Work out the finished part from the listing and answer in its coordinate system (mm). A direction names the side the tool comes from. Round coordinates to 2 decimals unless told otherwise and drop trailing zeros. Loops run counter-clockwise (first coordinate to the right, second up) from the corner with the lowest first, then second, coordinate; pieces in that order, holes last.
```python
from build123d import *

# Parameters (mm, degrees)
BOSS_EXTRUDE1_DEPTH = 12
CUT_EXTRUDE1_REACH  = 94.569
SKETCH2_R           = 3


with BuildPart() as part:
    # Sketch1 → Boss-Extrude1 (new body)
    with BuildSketch(Plane(origin=(0, 0, 0), x_dir=(1, 0, 0), z_dir=(0, 1, 0))):
        Polygon((-30, -30), (-45, -45), (-45, -80), (45, -80), (45, -45), (30, -30), (30, 30), (-30, 30), align=None)
    extrude(amount=BOSS_EXTRUDE1_DEPTH)

    # Sketch2 → Cut-Extrude1 (cut, up to next)
    with BuildSketch(Plane(origin=(0, 12, 0), x_dir=(1, 0, 0), z_dir=(0, 1, 0)), mode=Mode.PRIVATE) as cut_extrude1_sk1:
        with Locations(Location((-24, 20, 0), (0, 0, 270))):
            Circle(SKETCH2_R)
    cut_extrude1_tool1 = extrude(cut_extrude1_sk1.sketch, amount=-CUT_EXTRUDE1_REACH, mode=Mode.PRIVATE) & part.part
    # Sketch2 → Cut-Extrude1 (cut, up to next)
    with BuildSketch(Plane(origin=(0, 12, 0), x_dir=(1, 0, 0), z_dir=(0, 1, 0)), mode=Mode.PRIVATE) as cut_extrude1_sk2:
        with Locations(Location((-24, -20, 0), (0, 0, 270))):
            Circle(SKETCH2_R)
    cut_extrude1_tool2 = extrude(cut_extrude1_sk2.sketch, amount=-CUT_EXTRUDE1_REACH, mode=Mode.PRIVATE) & part.part
    # Sketch2 → Cut-Extrude1 (cut, up to next)
    with BuildSketch(Plane(origin=(0, 12, 0), x_dir=(1, 0, 0), z_dir=(0, 1, 0)), mode=Mode.PRIVATE) as cut_extrude1_sk3:
        with Locations(Location((24, 20, 0), (0, 0, 270))):
            Circle(SKETCH2_R)
    cut_extrude1_tool3 = extrude(cut_extrude1_sk3.sketch, amount=-CUT_EXTRUDE1_REACH, mode=Mode.PRIVATE) & part.part
    # Sketch2 → Cut-Extrude1 (cut, up to next)
    with BuildSketch(Plane(origin=(0, 12, 0), x_dir=(1, 0, 0), z_dir=(0, 1, 0)), mode=Mode.PRIVATE) as cut_extrude1_sk4:
        with Locations(Location((24, -20, 0), (0, 0, 270))):
            Circle(SKETCH2_R)
    cut_extrude1_tool4 = extrude(cut_extrude1_sk4.sketch, amount=-CUT_EXTRUDE1_REACH, mode=Mode.PRIVATE) & part.part
    add(cut_extrude1_tool1.solids().sort_by_distance((-24, 12, -20))[0], mode=Mode.SUBTRACT)
    add(cut_extrude1_tool2.solids().sort_by_distance((-24, 12, 20))[0], mode=Mode.SUBTRACT)
    add(cut_extrude1_tool3.solids().sort_by_distance((24, 12, -20))[0], mode=Mode.SUBTRACT)
    add(cut_extrude1_tool4.solids().sort_by_distance((24, 12, 20))[0], mode=Mode.SUBTRACT)


solid = part.part
```
1. Find section D-D (z = -9). Write down the section's boundary in (x, y), then the cut area to 3 significant figures.
Answer key:
outline: (-30, 0) - (30, 0) - (30, 12) - (-30, 12) - close
area: 720 mm2
2. Find section B-B (x = 24). Write down the section's boundary in (y, z).
Answer key:
outline: (0, -30) - (12, -30) - (12, -23) - (0, -23) - close; (0, -17) - (12, -17) - (12, 17) - (0, 17) - close; (0, 23) - (12, 23) - (12, 80) - (0, 80) - close
3. Find section C-C (z = -20). Write down the section's boundary in (x, y).
Answer key:
outline: (-30, 0) - (-27, 0) - (-27, 12) - (-30, 12) - close; (-21, 0) - (21, 0) - (21, 12) - (-21, 12) - close; (27, 0) - (30, 0) - (30, 12) - (27, 12) - close
4. Determine the mould class of faces 3 (the face through (-24, 6, -23)), 4 (the face through (-1, 0, 24)), 5 (the face through (30, 6, 0)), 6 (the face through (-37, 6, 37)) for opening direction X: +X half, -X half, draft (parallel to the pull), parting line (faces both ways), or undercut.
Answer key:
face 3: undercut
face 4: draft
face 5: +X half
face 6: -X half
5. Given pin 1 (4 mm diameter, centred on x = 34.5, y = 2.5, fed in from -Z); pin 2 (3.5 mm diameter, centred on y = 6.5, z = -0.5, fed in from +X); pin 3 (3 mm diameter, centred on x = 31, z = 0, fed in from +Y), each flat-ended and moving along its own axis, determine where each tip first touches the part or whether it passes through.
Answer key:
pin 1: stops at z = 32.5
pin 2: stops at x = 30
pin 3: stops at y = 12
6. Which of the six approach directions +Z, -Z, +X, -X, +Y, -Y give full straight-line access (tool end or side, diameter ignored) to faces 1 (the face through (-24, 6, 17)), 2 (the face through (-30, 6, 0))?
Answer key:
face 1: +Y, -Y
face 2: -Z, -X, +Y, -Y
7. Find section A-A (y = 7.5). Write down the section's boundary in (x, z), then the cut area to 3 significant figures.
Answer key:
outline: (-45, 45) - (-30, 30) - (-30, -30) - (30, -30) - (30, 30) - (45, 45) - (45, 80) - (-45, 80) - close; hole circle Ø6 at (-24, -20); hole circle Ø6 at (-24, 20); hole circle Ø6 at (24, -20); hole circle Ø6 at (24, 20)
area: 7,760 mm2
8. Consider probe 1 along X at (y, z) = (4.75, 20); probe 2 along X at (y, z) = (3, -18); probe 3 along X at (y, z) = (11, -8). Determine where each line is inside the solid, lowest interval first.
Answer key:
probe 1: x = -30 to -27, -21 to 21, 27 to 30
probe 2: x = -30 to -26.24, -21.76 to 21.76, 26.24 to 30
probe 3: x = -30 to 30
